The listing builds one solid part. Answer for the finished solid, in the listing's coordinates (mm). Face numbers are marked on the shaded views. A direction names the side the tool comes from. Give positions to 0.01 mm unless a question says otherwise; leave off trailing zeros. Loops run counter-clockwise (first coordinate to the right, second up) from the corner with the lowest first, then second, coordinate; pieces in that order, holes last. Notation, with made-up numbers: (22, -9.5) - (57, -9.5) arc R31 ccw to (57, 18.5) - close; hole circle Ø9 at (-29.75, -13.75). An arc over 180 degrees is marked (long way). Write each question's results on one line, items separated by ' | '.
from build123d import *

# Parameters (mm, degrees)
CROQUIS1_R              = 3.9
SALIENTE_EXTRUIR1_DEPTH = 30
CROQUIS2_R              = 3.25
SALIENTE_EXTRUIR2_DEPTH = 5
CROQUIS3_R              = 1.7
SALIENTE_EXTRUIR3_DEPTH = 20
REDONDEO1_R             = 1


with BuildPart() as part:
    # Croquis1 → Saliente-Extruir1 (new body)
    with BuildSketch(Plane(origin=(0, 0, 0), x_dir=(1, 0, 0), z_dir=(0, 1, 0))):
        with Locations(Location((0, 0, 0), (0, 0, 270))):
            Circle(CROQUIS1_R)
    extrude(amount=SALIENTE_EXTRUIR1_DEPTH)

    # Croquis2 → Saliente-Extruir2 (add)
    with BuildSketch(Plane(origin=(0, 30, 0), x_dir=(1, 0, 0), z_dir=(0, 1, 0))):
        with Locations(Location((0, 0, 0), (0, 0, 270))):
            Circle(CROQUIS2_R)
    extrude(amount=SALIENTE_EXTRUIR2_DEPTH)

    # Croquis3 → Saliente-Extruir3 (add)
    with BuildSketch(Plane.XZ):
        with Locations(Location((0, 0, 0), (0, 0, 270))):
            Circle(CROQUIS3_R)
    extrude(amount=SALIENTE_EXTRUIR3_DEPTH)

    # Redondeo1
    # the kernel refuses this fillet: 1 mm, written as the material it adds along each edge
    with BuildSketch(Plane(origin=(0, 30, 0), x_dir=(0, 0, 1), z_dir=(-1, 0, 0))) as redondeo1_piece_1:
        with BuildLine():
            CenterArc((4.25, 0.9367497), REDONDEO1_R, 180, 69.512684885)
            Line((3.25, 0.9367497), (3.23, 0.9367497))
            Line((3.23, 0.9367497), (3.23, 0))
            Line((3.23, 0), (3.25, -0.02))
            ThreePointArc((3.25, -0.02), (3.575, -0.02), (3.893, -0.018734994))
            Line((3.893, -0.018734994), (3.9, 0))
        make_face()
    revolve(axis=Axis((0, 30, 0), (0, 1, 0)))


solid = part.part
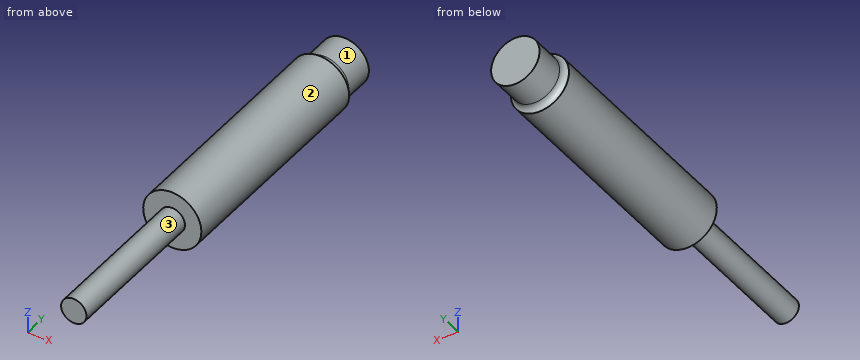
Item 1: A cutting plane is placed at A-A, the plane x = 0. Determine the outline of the cut face in (y, z), plus the area to 3 significant figures.
Values found:
outline: (-20, -1.7) - (0, -1.7) - (0, -3.9) - (30, -3.9) arc R1 cw to (30.94, -3.25) - (35, -3.25) - (35, 3.25) - (30.94, 3.25) arc R1 cw to (30, 3.9) - (0, 3.9) - (0, 1.7) - (-20, 1.7) - close | area: 335 mm²
Item 2: Find the intervals of material crossed by line 1 along Y through (x, z) = (-0.25, 1.75); line 2 along X through (y, z) = (1, -1); line 3 along Z through (x, y) = (3, 4), in increasing order. Write a range as [from, to].
Values found:
line 1: y = [0, 35] | line 2: x = [-3.77, 3.77] | line 3: z = [-2.49, 2.49]
Item 3: A cutting plane is placed at B-B, the plane z = 0. Determine the outline of the cut face in (x, y), plus the area to 3 significant figures.
Values found:
outline: (-3.9, 0) - (-1.7, 0) - (-1.7, -20) - (1.7, -20) - (1.7, 0) - (3.9, 0) - (3.9, 30) arc R1 cw to (3.25, 30.94) - (3.25, 35) - (-3.25, 35) - (-3.25, 30.94) arc R1 cw to (-3.9, 30) - close | area: 335 mm²
Item 4: A cutting plane is placed at C-C, the plane y = -7.5. Determine the outline of the cut face in (x, z), plus the area to 3 significant figures.
Values found:
outline: circle Ø3.4 at (0, 0) | area: 9.08 mm²
Item 5: For the marked faces 1, 2 and 3, determine the directions among +Z, -Z, +X, -X, +Y, -Y from which every point of the face is accessible in a straight line to the end or side of a thin tool.
Values found:
face 1: +Y | face 2: +Y, -Y | face 3: -Y
Item 6: Flat-ended cylindrical pins translate along their axes: P1, Ø4, axis at x = 0.5, z = 2, coming from the -Y side; P2, Ø2, axis at x = 0.5, z = 3, coming from the -Y side. Find the tip coordinate at first contact, or state that the pin passes through.
Values found:
P1: stops at y = -20 | P2: stops at y = 0
